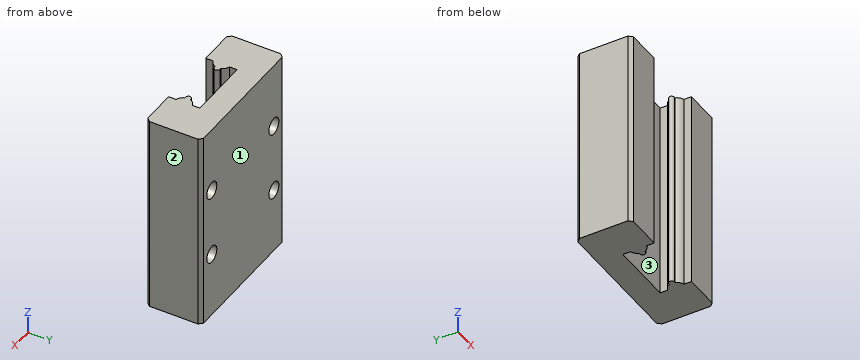
from build123d import *

# Parameters (mm, degrees)
EXTRUDE_1_DEPTH     = 28.9
SKETCH_2_R          = 1.2
CUT_EXTRUDE_1_DEPTH = 5


with BuildPart() as part:
    # 草图1 → 凸台-拉伸1 (new body)
    with BuildSketch(Plane.XY):
        with BuildLine():
            Line((0, 0.5), (0, 7.5))
            Line((0, 7.5), (0.5, 8))
            Line((0.5, 8), (19.5, 8))
            Line((19.5, 8), (20, 7.5))
            Line((20, 7.5), (20, 0.5))
            Line((20, 0.5), (19.5, 0))
            Line((19.5, 0), (14.5, 0))
            Line((14.5, 0), (14.5, 1.088104996))
            ThreePointArc((14.5, 1.088104996), (13.989243177, 1.365311708), (13.66862915, 1.85))
            Line((13.66862915, 1.85), (13.5, 1.85))
            ThreePointArc((13.5, 1.85), (13.1, 2.25), (13.5, 2.65))
            Line((13.5, 2.65), (13.66862915, 2.65))
            ThreePointArc((13.66862915, 2.65), (13.989243177, 3.134688292), (14.5, 3.411895004))
            Line((14.5, 3.411895004), (14.5, 4.5))
            Line((14.5, 4.5), (5.5, 4.5))
            Line((5.5, 4.5), (5.5, 3.411895004))
            ThreePointArc((5.5, 3.411895004), (6.010756823, 3.134688292), (6.33137085, 2.65))
            Line((6.33137085, 2.65), (6.5, 2.65))
            ThreePointArc((6.5, 2.65), (6.9, 2.25), (6.5, 1.85))
            Line((6.5, 1.85), (6.33137085, 1.85))
            ThreePointArc((6.33137085, 1.85), (6.010756823, 1.365311708), (5.5, 1.088104996))
            Line((5.5, 1.088104996), (5.5, 0))
            Line((5.5, 0), (0.5, 0))
            Line((0.5, 0), (0, 0.5))
        make_face()
    extrude(amount=EXTRUDE_1_DEPTH)

    # 草图2 → 切除-拉伸1 (cut)
    with BuildSketch(Plane(origin=(0, 8, 0), x_dir=(1, 0, 0), z_dir=(0, 1, 0))):
        with Locations(Location((2.5, -19.45, 0), (0, 0, 270))):
            Circle(SKETCH_2_R)
        with Locations(Location((2.5, -9.45, 0), (0, 0, 270))):
            Circle(SKETCH_2_R)
        with Locations(Location((17.5, -9.45, 0), (0, 0, 270))):
            Circle(SKETCH_2_R)
        with Locations(Location((17.5, -19.45, 0), (0, 0, 270))):
            Circle(SKETCH_2_R)
    extrude(amount=-CUT_EXTRUDE_1_DEPTH, mode=Mode.SUBTRACT)


solid = part.part
The listing builds one solid part. Answer for the finished solid, in the listing's coordinates (mm). Face numbers are marked on the shaded views. Coordinates: 2 decimals unless noted, no trailing zeros. Write each loop counter-clockwise with the first axis right and the second up, starting at its lowest first coordinate (ties: lowest second). Pieces come first, ordered by that corner, then holes. Notation, with made-up numbers: (-26, -3.75) - (8, -3.75) arc R24 ccw to (8, 34.25) - close; hole circle Ø8 at (44.25, 63). An arc over 180 degrees is marked (long way). Return JSON: item names as keys, results as strings.
1. For a pull along X with two mould halves and no side action, classify the marked faces 1, 2 and 3 as +X half, -X half, draft (parallel to the pull), parting line (faces both ways), or undercut.
Final values:
{"face 1": "draft", "face 2": "+X half", "face 3": "undercut"}
2. The part is cut by section A-A on y = 2.25. Determine the outline of the cut face in (x, z), then the cut area to 3 significant figures.
Final values:
{"outline": "(0, 0) - (6.9, 0) - (6.9, 28.9) - (0, 28.9) - close; (13.1, 0) - (20, 0) - (20, 28.9) - (13.1, 28.9) - close", "area": "399 mm^2"}
3. Consider line 1 along X through (y, z) = (7, 9.45); line 2 along X through (y, z) = (4.4, 9.45); line 3 along X through (y, z) = (3.5, 27.25). Determine where each line is inside the solid, lowest interval first.
Final values:
{"line 1": "0 to 1.3, 3.7 to 16.3, 18.7 to 20", "line 2": "0 to 1.3, 3.7 to 5.5, 14.5 to 16.3, 18.7 to 20", "line 3": "0 to 5.5, 14.5 to 20"}
4. The part is cut by section D-D on x = 2.5. Determine the outline of the cut face in (y, z), then the cut area to 3 significant figures.
Final values:
{"outline": "(0, 0) - (8, 0) - (8, 8.25) - (3, 8.25) - (3, 10.65) - (8, 10.65) - (8, 18.25) - (3, 18.25) - (3, 20.65) - (8, 20.65) - (8, 28.9) - (0, 28.9) - close", "area": "207 mm^2"}
5. The part is cut by section B-B on z = 2.5. Determine the outline of the cut face in (x, y).
Final values:
{"outline": "(0, 0.5) - (0.5, 0) - (5.5, 0) - (5.5, 1.09) arc R1.2 ccw to (6.33, 1.85) - (6.5, 1.85) arc R0.4 ccw to (6.5, 2.65) - (6.33, 2.65) arc R1.2 ccw to (5.5, 3.41) - (5.5, 4.5) - (14.5, 4.5) - (14.5, 3.41) arc R1.2 ccw to (13.67, 2.65) - (13.5, 2.65) arc R0.4 ccw to (13.5, 1.85) - (13.67, 1.85) arc R1.2 ccw to (14.5, 1.09) - (14.5, 0) - (19.5, 0) - (20, 0.5) - (20, 7.5) - (19.5, 8) - (0.5, 8) - (0, 7.5) - close"}
6. The part is cut by section C-C on y = 7. Determine the outline of the cut face in (x, z), then the cut area to 3 significant figures.
Final values:
{"outline": "(0, 0) - (20, 0) - (20, 28.9) - (0, 28.9) - close; hole circle Ø2.4 at (2.5, 9.45); hole circle Ø2.4 at (2.5, 19.45); hole circle Ø2.4 at (17.5, 9.45); hole circle Ø2.4 at (17.5, 19.45)", "area": "560 mm^2"}
7. Each of these flat-tipped pins is pushed along its axis until it touches: pin 1 Ø1.9 at (x, z) = (17.5, 9.45) entering from +Y; pin 2 Ø1.9 at (x, z) = (2.5, 9.45) entering from -Y. Where does it stop, or does it pass through?
Final values:
{"pin 1": "y = 3", "pin 2": "y = 0"}
